from build123d import *

# Parameters (mm, degrees)
F1_DEPTH = 177.8
F3_DEPTH = 73.025


with BuildPart() as f1:
    # F0 (on Right) → F1 (new body, symmetric)
    with BuildSketch(Plane.YZ):
        with BuildLine():
            Line((0, -12.7), (0, -152.4))
            Line((0, -152.4), (5.0270461919, -152.4))
            Line((5.0270461919, -152.4), (5.0270461919, -12.7))
            ThreePointArc((5.0270461919, -12.7), (7.2744023306, -7.2744023306), (12.7, -5.0270461919))
            Line((12.7, -5.0270461919), (50.8, -5.0270461919))
            Line((50.8, -5.0270461919), (50.8, 0))
            Line((50.8, 0), (12.7, 0))
            ThreePointArc((12.7, 0), (3.7197438789, -3.7197438789), (0, -12.7))
        make_face()
    extrude(amount=F1_DEPTH, both=True)

    # F2 (on face) → F3 (join)
    with BuildSketch(Plane.XZ):
        with BuildLine():
            Line((-108.298035616, -65.0875), (-107.95, -60.325))
            Line((-107.95, -60.325), (-161.925, -60.325))
            ThreePointArc((-161.925, -60.325), (-168.6601920908, -63.1148079092), (-171.45, -69.85))
            Line((-171.45, -69.85), (-171.45, -146.05))
            Line((-171.45, -146.05), (-166.6875, -146.05))
            Line((-166.6875, -146.05), (-166.6875, -69.85))
            ThreePointArc((-166.6875, -69.85), (-165.2925960454, -66.4824039546), (-161.925, -65.0875))
            Line((-161.925, -65.0875), (-108.298035616, -65.0875))
        make_face()
    extrude(amount=F3_DEPTH)

    # F4: F1 across plane


with BuildPart() as f1_1:
    add(f1.part)
    add(f1.part.mirror(Plane.YZ))


solid = f1_1.part
For this review, take the finished solid that the model builds, in its own axes (mm). A direction names the side the tool comes from. Round coordinates to 2 decimals unless told otherwise and drop trailing zeros. Write each loop counter-clockwise with the first axis right and the second up, starting at its lowest first coordinate (ties: lowest second). Pieces come first, ordered by that corner, then holes. Notation, with made-up numbers: (23.25, -10) -> (76.25, -10) arc R21 cw to (76.25, 23) -> close; hole circle Ø7 at (-21.5, 81). An arc over 180 degrees is marked (long way). Put each result on its own line as item: value.
Q1. To check wall thickness, follow L1, parallel to X at y = -67.5, z = -125.5; L2, parallel to Y at x = 90, z = -72; L3, parallel to Y at x = -145, z = -61 (3 decimals). State the ranges of each line that lie inside material, in increasing order. Write a range as [from, to].
Determined:
L1: x = [-171.45, -166.69], [166.69, 171.45]
L2: y = [0, 5.03]
L3: y = [-73.025, 5.027]
Q2. Machinability: for faces 4 (the cylindrical face through (-168.586, -36.001, -63.041)), 5 (the flat face through (2, 5.027, -84)), 6 (the flat face through (171.45, -36, -107)), 7 (the flat face through (-135, -36, -60.325)), 8 (the flat face through (-135, -36, -65.088)), which of the approach directions +Z, -Z, +X, -X, +Y, -Y give a long, thin tool a straight path to every point of the face, cutting with its end or side? Answer none if there is none.
Determined:
face 4: +Z, -X, -Y
face 5: -Z, +X, -X, +Y
face 6: +Z, -Z, +X, -Y
face 7: +Z, +X, -X, -Y
face 8: -Z, -Y
Q3. Consider section C-C on x = 146. State the section outline as (y, z) points (1 decimal).
Determined:
outline: (-73, -65.1) -> (0, -65.1) -> (0, -152.4) -> (5, -152.4) -> (5, -12.7) arc R7.7 cw to (12.7, -5) -> (50.8, -5) -> (50.8, 0) -> (12.7, 0) arc R12.7 ccw to (0, -12.7) -> (0, -60.3) -> (-73, -60.3) -> close
Q4. Consider section D-D on y = 31. State the section outline as (x, z) points, and give its area (3 significant figures).
Determined:
outline: (-177.8, -5.03) -> (177.8, -5.03) -> (177.8, 0) -> (-177.8, 0) -> close
area: 1,790 mm^2
Q5. Clearance check with flat-ended pins moving along their axes: pin 1 Ø16 at (x, y) = (-131.5, -26) entering from +Z (3 decimals); pin 2 Ø6 at (y, z) = (-60, -100.5) entering from +X; pin 3 Ø22 at (y, z) = (-52, -107) entering from -X. State where each tip first meets the part, or that it passes through.
Determined:
pin 1: stops at z = -60.325
pin 2: stops at x = 171.45
pin 3: stops at x = -171.45
Q6. The part is to be moulded in two halves that separate along X. For faces 1 (the flat face through (-166.688, -36, -108)), 2 (the cylindrical face through (168.586, -36.001, -63.041)), 3 (the flat face through (-171.45, -36, -107)), say which applies: released by +X, released by -X, zero draft, split by the parting line, or undercut.
Determined:
face 1: undercut
face 2: released by +X
face 3: released by -X
